```python
from build123d import *

# Parameters (mm, degrees)
SKETCH1_W           = 38.1
SKETCH1_H           = 25.4
BOSS_EXTRUDE1_DEPTH = 50.8
CUT_EXTRUDE1_DEPTH  = 12.7


with BuildPart() as part:
    # Sketch1 → Boss-Extrude1 (new body)
    with BuildSketch(Plane.XY):
        Rectangle(SKETCH1_W, SKETCH1_H)
    extrude(amount=BOSS_EXTRUDE1_DEPTH)

    # Sketch2 → Cut-Extrude1 (cut)
    with BuildSketch(Plane(origin=(0, 12.7, 0), x_dir=(1, 0, 0), z_dir=(0, 1, 0))):
        with BuildLine():
            Line((19.05, -8.255), (0, -8.255))
            ThreePointArc((0, -8.255), (-9.525, -17.78), (0, -27.305))
            Line((0, -27.305), (19.05, -27.305))
            Line((19.05, -27.305), (19.05, -8.255))
        make_face()
    extrude(amount=-CUT_EXTRUDE1_DEPTH, mode=Mode.SUBTRACT)


solid = part.part
```
Design review of the part built by this model. Coordinates are the model's own, in mm. A direction names the side the tool comes from. Round coordinates to 2 decimals unless told otherwise and drop trailing zeros. Order: outer loops, then holes, each group sorted by start corner. A loop starts at its lowest first (then second) coordinate and runs counter-clockwise, first axis right, second up. Notation, with made-up numbers: (-39.5, 0.25) - (-23.5, 0.25) arc R29 cw to (-23.5, 21.25) - close; hole circle Ø5 at (63.25, 3). An arc over 180 degrees is marked (long way). Return JSON: item names as keys, results as strings.
Q1. Consider section C-C on x = -6.5. Write out the cut boundary in (y, z).
Computed values:
{"outline": "(-12.7, 0) - (12.7, 0) - (12.7, 10.82) - (0, 10.82) - (0, 24.74) - (12.7, 24.74) - (12.7, 50.8) - (-12.7, 50.8) - close"}
Q2. Consider section A-A on x = 6. Write out the cut boundary in (y, z) (3 decimals).
Computed values:
{"outline": "(-12.7, 0) - (12.7, 0) - (12.7, 8.255) - (0, 8.255) - (0, 27.305) - (12.7, 27.305) - (12.7, 50.8) - (-12.7, 50.8) - close"}
Q3. Machinability: for faces 1 (the flat face through (0, 12.7, 31)), 2 (the cylindrical face through (-9.523, 6.439, 17.571)), which of the approach directions +Z, -Z, +X, -X, +Y, -Y give a long, thin tool a straight path to every point of the face, cutting with its end or side? Answer none if there is none.
Computed values:
{"face 1": "+Z, -Z, +X, -X, +Y", "face 2": "+X, +Y"}
Q4. The part is to be moulded in two halves that separate along Z. For faces 3 (the flat face through (0, 0, 0)), 4 (the flat face through (10, 6, 8.255)), 5 (the flat face through (0, 0, 50.8)), say which applies: pulls with the +Z half, pulls with the -Z half, needs draft (parallel to the pull), parting line crosses it, or undercut.
Computed values:
{"face 3": "pulls with the -Z half", "face 4": "undercut", "face 5": "pulls with the +Z half"}
Q5. Wall thickness on L1, parallel to Z at x = 15.5, y = 9.25 (3 decimals); L2, parallel to Y at x = 2.5, z = 20; L3, parallel to Z at x = -1.5, y = 11.75: over which ranges is each line inside the solid? List them lowest first. Write a range as [from, to].
Computed values:
{"L1": "z = [0, 8.255], [27.305, 50.8]", "L2": "y = [-12.7, 0]", "L3": "z = [0, 8.37], [27.19, 50.8]"}
Q6. Consider section B-B on z = 17.78. Write out the cut boundary in (x, y) (3 decimals), plus the area to 3 significant figures.
Computed values:
{"outline": "(-19.05, -12.7) - (19.05, -12.7) - (19.05, 0) - (-9.525, 0) - (-9.525, 12.7) - (-19.05, 12.7) - close", "area": "605 mm2"}
